Autodesk Inventor part; units mm, degrees
ref_plane "YZ Plane" through (0, 0, 0) normal (1, 0, 0) x (0, 1, 0)
ref_plane "XZ Plane" through (0, 0, 0) normal (0, 1, 0) x (-1, 0, 0)
ref_plane "XY Plane" through (0, 0, 0) normal (0, 0, 1) x (1, 0, 0)
sketch "Sketch1" plane through (0, 0, 0) normal (0, 0, 1) x (1, 0, 0)
  line L0 (0, 0) -> (88.9, 0)
  line L1 (88.9, 0) -> (88.9, -63.5)
  line L2 (88.9, -63.5) -> (0, -63.5)
  line L3 (0, -63.5) -> (0, 0)
  line L4 (6.985, -8.255) -> (81.915, -8.255)
  line L5 (81.915, -8.255) -> (81.915, -55.245)
  line L6 (81.915, -55.245) -> (6.985, -55.245)
  line L7 (6.985, -55.245) -> (6.985, -8.255)
  dimension "d0" = 88.9
  dimension "d1" = 63.5
  dimension "d2" = 8.255
  dimension "d3" = 8.255
  dimension "d4" = 6.985
  dimension "d5" = 6.985
extrude "Extrusion1" add sketch "Sketch1" along normal blind 5.08
sketch "Sketch2" plane through (0, 0, 5.08) normal (0, 0, 1) x (1, 0, 0)
  circle A0 centre (3.4925, -12.7) radius 3.175
  circle A1 centre (3.4925, -50.8) radius 3.175
  circle A2 centre (85.4075, -50.8) radius 3.175
  circle A3 centre (85.4075, -12.7) radius 3.175
  line L0 (88.9, 0) -> (0, 0)
  line L1 (0, -63.5) -> (88.9, -63.5)
  line L2 (0, 0) -> (0, -63.5)
  line L3 (81.915, -8.255) -> (81.915, -55.245)
  circle A4 centre (85.4075, -50.8) radius 1.905
  circle A5 centre (85.4075, -12.7) radius 1.905
  circle A6 centre (3.4925, -50.8) radius 1.905
  circle A7 centre (3.4925, -12.7) radius 1.905
  dimension "d8" = 6.35
  dimension "d9" = 6.35
  dimension "d10" = 6.35
  dimension "d11" = 6.35
  dimension "d12" = 12.7
  dimension "d13" = 12.7
  dimension "d14" = 12.7
  dimension "d15" = 12.7
  dimension "d16" = 3.4925
  dimension "d17" = 3.4925
  dimension "d18" = 3.81
extrude "Extrusion2" add sketch "Sketch2" along normal blind 7.62
sketch "Sketch3" plane through (0, 0, 0) normal (0, 0, -1) x (-1, 0, 0)
  line L0 (0, 7.62) -> (0, -71.12)
  line L1 (-88.9, -71.12) -> (-88.9, 7.62)
  line L2 (0, 0) -> (-88.9, 0)
  line L3 (-88.9, -63.5) -> (0, -63.5)
  line L4 (-88.9, 0) -> (-88.9, -63.5)
  line L5 (0, -63.5) -> (0, 0)
  line L6 (-35.56, 0) -> (-35.56, 7.62)
  line L7 (-53.34, 7.62) -> (-53.34, 0)
  line L8 (0, -63.5) -> (-88.9, -63.5)
  line L9 (-53.34, -63.5) -> (-53.34, -71.12)
  line L10 (-35.56, -63.5) -> (-35.56, -71.12)
  line L11 (-88.9, 7.62) -> (-53.34, 7.62)
  line L12 (-35.56, 7.62) -> (0, 7.62)
  line L13 (0, -71.12) -> (-35.56, -71.12)
  line L14 (-53.34, -71.12) -> (-88.9, -71.12)
  point P0 (-88.9, -31.75)
  point P1 (0, -31.75)
  dimension "d23" = 35.56
  dimension "d24" = 35.56
extrude "Extrusion3" add sketch "Sketch3" along normal blind 1.905
sketch "Sketch4" plane through (0, 0, 0) normal (0, 0, 1) x (1, 0, 0)
  line L0 (6.985, -8.255) -> (81.915, -8.255)
  line L1 (81.915, -8.255) -> (81.915, -55.245)
  line L2 (81.915, -55.245) -> (6.985, -55.245)
  line L3 (6.985, -55.245) -> (6.985, -8.255)
  point P0 (0, 0)
extrude "Extrusion4" cut sketch "Sketch4" against normal blind 1.905
sketch "Sketch5" plane through (0, 0, -1.905) normal (0, 0, -1) x (-1, 0, 0)
  line L0 (0, -63.5) -> (-88.9, -63.5)
  line L1 (-53.34, 0) -> (-35.56, 0)
  line L2 (-35.56, 0) -> (-35.56, -63.5)
  line L3 (-35.56, -63.5) -> (-53.34, -63.5)
  line L4 (-53.34, -63.5) -> (-53.34, 0)
  point P0 (0, 0)
  dimension "d29" = 17.78
extrude "Extrusion5" cut sketch "Sketch5" against normal blind 3.175
sketch "Sketch6" plane through (85.4075, -12.7, 12.7) normal (0, 0, 1) x (1, 0, 0)
  circle A0 centre (0, 0) radius 1.905
  circle A1 centre (-81.915, 0) radius 1.905
  circle A2 centre (-81.915, 0) radius 1.905
  circle A3 centre (0, -38.1) radius 1.905
  circle A4 centre (0, -38.1) radius 1.905
  circle A5 centre (-81.915, -38.1) radius 1.905
  circle A6 centre (-81.915, -38.1) radius 1.905
  point P0 (-85.4075, 12.7)
extrude "Extrusion6" cut sketch "Sketch6" against normal blind 25.4
properties part number "Heatsink al base" material "Aluminum 6061"
For this review, take the finished solid that the model builds, in its own axes (mm). A direction names the side the tool comes from. Coordinates: 2 decimals unless noted, no trailing zeros. Write each loop counter-clockwise with the first axis right and the second up, starting at its lowest first coordinate (ties: lowest second). Pieces come first, ordered by that corner, then holes. Notation, with made-up numbers: (11, 84.5) - (17, 84.5) arc R25 cw to (17, 102.5) - close; hole circle Ø9 at (13, 63). An arc over 180 degrees is marked (long way). Answer in a Markdown table with one row per item. Add a question column.
Q1. We need section C-C, the plane y = -23. State the section outline as (x, z) points (3 decimals).
Q2. For probe 1 along Y at (x, z) = (29, 3) (3 decimals); probe 2 along X at (y, z) = (-40, 4.5) (3 decimals); probe 3 along Y at (x, z) = (4, 3), list the stretches that pass through material, from the lowest coordinate up.
Q3. We need section A-A, the plane x = 26. State the section outline as (y, z) points (3 decimals).
Q4. For P1, Ø2, axis at x = 34.5, z = 8, coming from the +Y side; P2, Ø4, axis at x = 48, y = -2.5, coming from the -Z side; P3, Ø8.5, axis at x = 62.5, y = 4, coming from the +Z side; P4, Ø6, axis at x = 48.5, z = -0.5, coming from the +Y side, all flat-tipped, find the tip position at first contact; note any pin that passes through.
Q5. Draft analysis for pull direction Y (two halves, no side actions). For faces 1 (the flat face through (18, 4, 0)), 2 (the flat face through (6.985, -32, 2)), 3 (the flat face through (71, 7.62, -1)), state which applies: +Y half, -Y half, draft (parallel to the pull), parting line (faces both ways), or undercut.
Q6. We need section D-D, the plane y = -62.5. State the section outline as (x, z) points (3 decimals).
Q7. Tool access review of faces 4 (the flat face through (45, -55.245, 2)), 5 (the cylindrical face through (4.958, -9.883, 8.837)), 6 (the flat face through (53.34, -62, -1)), 7 (the flat face through (71, 4, 0)): name each direction out of +Z, -Z, +X, -X, +Y, -Y from which nothing blocks a thin tool from reaching the whole face with its end or side.
Q8. We need section B-B, the plane y = -50.8. Count the separate pieces of the cut face and the enclosed holes in it, and give its area (3 significant figures).
Answer list:
| question | item | result |
|---|---|---|
| 1 | outline | (0, -1.905) - (6.985, -1.905) - (6.985, 5.08) - (0, 5.08) - close; (81.915, -1.905) - (88.9, -1.905) - (88.9, 5.08) - (81.915, 5.08) - close |
| 2 | probe 1 | y = -63.5 to -55.245, -8.255 to 0 |
| 2 | probe 2 | x = 0 to 6.985, 81.915 to 88.9 |
| 2 | probe 3 | y = -63.5 to -52.64, -48.96 to -14.54, -10.86 to 0 |
| 3 | outline | (-71.12, -1.905) - (-55.245, -1.905) - (-55.245, 5.08) - (-63.5, 5.08) - (-63.5, 0) - (-71.12, 0) - close; (-8.255, -1.905) - (7.62, -1.905) - (7.62, 0) - (0, 0) - (0, 5.08) - (-8.255, 5.08) - close |
| 4 | P1 | passes through |
| 4 | P2 | stops at z = 1.27 |
| 4 | P3 | stops at z = 5.08 |
| 4 | P4 | stops at y = 0 |
| 5 | face 1 | draft |
| 5 | face 2 | undercut |
| 5 | face 3 | +Y half |
| 6 | outline | (0, -1.905) - (35.56, -1.905) - (35.56, 1.27) - (53.34, 1.27) - (53.34, -1.905) - (88.9, -1.905) - (88.9, 5.08) - (0, 5.08) - close |
| 7 | face 4 | +Z, -Z |
| 7 | face 5 | +Z |
| 7 | face 6 | -Z, +Y, -Y |
| 7 | face 7 | +Z, +X, -X, +Y |
| 8 | separate pieces | 4 |
| 8 | enclosed holes | 0 |
| 8 | area | 83.1 mm2 |
